Part model, mm, in its own coordinate system. A direction names the side the tool comes from. Coordinates: 2 decimals unless noted, no trailing zeros. Order: outer loops, then holes, each group sorted by start corner. A loop starts at its lowest first (then second) coordinate and runs counter-clockwise, first axis right, second up.
1) Mould opens along Y. For faces 1 (the flat face through (3.642, -2.142, -17.072)), 2 (the flat face through (16.5, 2.2, 2.3)), 3 (the cylindrical face through (-8.935, -24.241, -17.854)) say: +Y half, -Y half, draft (parallel to the pull), parting line (faces both ways), or undercut.
2) Cut at D-D (x = -0.75). List the corners of the cut face in (y, z) (3 decimals), and give its area (3 significant figures).
3) Pin check, flat tips, straight feed: pin 1 Ø7 at (x, y) = (-1.5, -22) entering from +Z; pin 2 Ø1.7 at (x, z) = (15, -0.5) entering from +Y; pin 3 Ø7 at (x, y) = (0, -20.5) entering from +Z. Stop position of each tip, or through.
4) Cut at B-B (x = 8.75). List the corners of the cut face in (y, z) (3 decimals), and give its area (3 significant figures).
5) Wall check: L1, parallel to Y at x = 0, z = -20.65; L2, parallel to Z at x = -10.25, y = 0 (3 decimals); L3, parallel to Y at x = 1.75, z = -16.5 (3 decimals). Give the ranges that are in metal, low to high.
6) Cut at A-A (z = -16). Give the number of separate pieces and of enclosed holes in the cut face, and give its area (3 significant figures).
7) Cut at C-C (y = -21). List the corners of the cut face in (x, z).
8) Tool access for faces 4 (the flat face through (0, 4.225, -17)), 5 (the flat face through (12.5, -1, -11)), 6 (the flat face through (-10, -13, -5)): list every direction of +Z, -Z, +X, -X, +Y, -Y with a clear straight run to the whole face (end or side of a thin tool).
```python
from build123d import *

# Parameters (mm, degrees)
F0_R      = 2.125
F1_DEPTH  = 12.5
F2_W      = 15.4
F2_H      = 26
F3_DEPTH  = 28.101
F4_R      = 2.25
F5_DEPTH  = 25
F7_DEPTH  = 4
F8_R      = 12.49999
F9_SIZE   = 5
F10_R     = 5
F11_DEPTH = 4
F12_SIZE  = 3.99999


# Not quite as in the source:
# - a fillet or chamfer is up to 0.001 mm smaller than in the source, because OpenCascade refuses the exact size
# - a feature names something its author has since deleted; it is built from what else it names


with BuildPart() as f1:
    # F0 (on Right) → F1 (new body, symmetric)
    with BuildSketch(Plane.YZ):
        with BuildLine():
            Line((13, -15.1), (13, 0))
            ThreePointArc((13, 0), (0, 13), (-13, 0))
            Line((-13, 0), (-13, -15.1))
            Line((-13, -15.1), (-28, -15.1))
            Line((-28, -15.1), (-28, -21.1))
            Line((-28, -21.1), (0, -21.1))
            Line((0, -21.1), (13, -21.1))
            Line((13, -21.1), (13, -15.1))
        make_face()
        Circle(F0_R, mode=Mode.SUBTRACT)
    extrude(amount=F1_DEPTH, both=True)

    # F2 (on face) → F3 (cut, through all)
    with BuildSketch(Plane.XY.offset(-15.1)):
        Rectangle(F2_W, F2_H)
    extrude(amount=F3_DEPTH, mode=Mode.SUBTRACT)

    # F4 (on face) → F5 (cut)
    with BuildSketch(Plane.XY.offset(-15.1)):
        with Locations((0, -20.5)):
            Circle(F4_R)
        Circle(F4_R)
    extrude(amount=-F5_DEPTH, mode=Mode.SUBTRACT)

    # F6 (on face) → F7 (cut)
    with BuildSketch(Plane.XY.offset(-15.1)):
        Polygon((-4.8786097747, -20.5), (-2.4393048873, -24.725), (2.4393048873, -24.725), (4.8786097747, -20.5), (2.4393048873, -16.275), (-2.4393048873, -16.275), align=None)
        Polygon((2.4393048873, 4.225), (-2.4393048873, 4.225), (-4.8786097747, 0), (-2.4393048873, -4.225), (2.4393048873, -4.225), (4.8786097747, 0), align=None)
    extrude(amount=-F7_DEPTH, mode=Mode.SUBTRACT)

    # F8 (radius 12.5 in the source; OpenCascade refuses exactly that, so slightly less here)
    f8_edges = [f1.edges().sort_by_distance(p)[0] for p in [
        (-12.5, -28, -18.1),
        (12.5, -28, -18.1),
    ]]
    fillet(f8_edges, radius=F8_R)

    # F9
    f9_edges = [f1.edges().sort_by_distance(p)[0] for p in [
        (-10.1, -13, -15.1),
        (10.1, -13, -15.1),
        (10.1, 13, 0),
        (-10.1, 13, 0),
    ]]
    chamfer(f9_edges, length=F9_SIZE)

    # F10 (on face) → F11 (join)
    with BuildSketch(Plane.YZ.offset(12.5)):
        Circle(F10_R)
        Polygon((0, 3.3746123234), (2.9225, 1.6873061617), (2.9225, -1.6873061617), (0, -3.3746123234), (-2.9225, -1.6873061617), (-2.9225, 1.6873061617), align=None, mode=Mode.SUBTRACT)
    extrude(amount=F11_DEPTH)

    # F12 (size 4 in the source; OpenCascade refuses exactly that, so slightly less here)
    f12_edges = [f1.edges().sort_by_distance(p)[0] for p in [
        (12.5, -5, 0),
    ]]
    chamfer(f12_edges, length=F12_SIZE)


solid = f1.part
```
Geometry check:
1. face 1: undercut
1. face 2: draft
1. face 3: -Y half
2. outline: (-27.977, -21.1) - (-22.621, -21.1) - (-22.621, -19.1) - (-24.725, -19.1) - (-24.725, -15.1) - (-27.977, -15.1) - close; (-18.379, -21.1) - (-2.121, -21.1) - (-2.121, -19.1) - (-4.225, -19.1) - (-4.225, -15.1) - (-16.275, -15.1) - (-16.275, -19.1) - (-18.379, -19.1) - close; (2.121, -21.1) - (13, -21.1) - (13, -15.1) - (4.225, -15.1) - (4.225, -19.1) - (2.121, -19.1) - close
2. area: 161 mm2
3. pin 1: stops at z = -15.1
3. pin 2: stops at y = 7.33
3. pin 3: stops at z = -19.1
4. outline: (-24.427, -21.1) - (13, -21.1) - (13, 0) arc R13 ccw to (-13, 0) - (-13, -10.1) - (-18, -15.1) - (-24.427, -15.1) - close; hole circle Ø4.25 at (0, 0)
4. area: 881 mm2
5. L1: y = -28 to -22.75, -18.25 to -2.25, 2.25 to 13
5. L2: z = -21.1 to -2.125, 2.125 to 13
5. L3: y = -27.877 to -24.725, -16.275 to -4.225, 4.225 to 13
6. separate pieces: 1
6. enclosed holes: 2
6. area: 834 mm2
7. outline: (-11.22, -21.1) - (-2.19, -21.1) - (-2.19, -19.1) - (-4.59, -19.1) - (-4.59, -15.1) - (-11.22, -15.1) - close; (2.19, -21.1) - (11.22, -21.1) - (11.22, -15.1) - (4.59, -15.1) - (4.59, -19.1) - (2.19, -19.1) - close
8. face 4: +Z
8. face 5: +X
8. face 6: +Z, +X, -X, -Y
